```python
from build123d import *

# Parameters (mm, degrees)
F1_DEPTH = 3


with BuildPart() as f1:
    # F0 (on Front) → F1 (new body)
    with BuildSketch(Plane.XZ):
        with BuildLine():
            Line((0, 272), (0, 0))
            Line((0, 0), (180, 0))
            Line((180, 0), (180, 70))
            add(Edge.make_bspline(
                [(215.824013933, 148.5454355016), (208.91407131, 143.3580070922), (174.748380555, 116.4051533787), (180.2117525716, 86.4379331497), (180, 70)],
                knots=[0, 0, 0, 0, 0.4976525843, 1, 1, 1, 1], degree=3))
            Line((215.824013933, 148.5454355016), (265, 184.6386813286))
            Line((265, 184.6386813286), (118, 272))
            Line((118, 272), (0, 272))
        make_face()
    extrude(amount=F1_DEPTH)


solid = f1.part
```
Geometry check sheet. Reference: the model listing, model coordinates, mm. Give positions to 0.01 mm unless a question says otherwise; leave off trailing zeros. Order: outer loops, then holes, each group sorted by start corner. A loop starts at its lowest first (then second) coordinate and runs counter-clockwise, first axis right, second up. Notation, with made-up numbers: (-35.75, -29) -> (14.25, -29) arc R21 cw to (14.25, 9) -> close; hole circle Ø2 at (-30, 78). An arc over 180 degrees is marked (long way). Write each question's results on one line, items separated by ' | '. Start each with the question number.
(1) Sectioned sample at B-B (x = 223). Enter the section's corners in (y, z).
(2) Gauge pin test, flat ends, axial feed: P1, Ø1.5, axis at y = -1, z = 180, coming from the -X side; P2, Ø0.9, axis at y = -2, z = 31, coming from the +X side. Record the tip position at first contact, or that the pin passes through.
(3) Sectioned sample at A-A (z = 59). Enter the section's corners in (x, y).
(4) Scan lines: line 1 (X direction, y = -0.55, z = 29); line 2 (X direction, y = -1.15, z = 235.5); line 3 (Z direction, x = 132.5, y = -0.2). Record each from-to range of solid material in increasing order.
Answer below:
1) outline: (-3, 153.81) -> (0, 153.81) -> (0, 209.6) -> (-3, 209.6) -> close
2) P1: x = 0 | P2: x = 180
3) outline: (0, -3) -> (180, -3) -> (180, 0) -> (0, 0) -> close
4) line 1: 0 to 180 | line 2: 0 to 179.42 | line 3: 0 to 263.38
